Read the model definition and answer for the solid it produces. Units are mm, in the model's axes. A direction names the side the tool comes from. Give positions to 0.01 mm unless a question says otherwise; leave off trailing zeros. Order: outer loops, then holes, each group sorted by start corner. A loop starts at its lowest first (then second) coordinate and runs counter-clockwise, first axis right, second up. Notation, with made-up numbers: (-21.5, -18.75) - (-5.5, -18.75) arc R30 ccw to (-5.5, 12.25) - close; hole circle Ø5 at (84.5, 84.25). An arc over 180 degrees is marked (long way). Write each question's results on one line, items separated by ' | '. Start each with the question number.
Q1. A tool of negligible diameter and unlimited length cuts with its end or side. For faces 1 (the face through (-25, -3, 2)), 2 (the face through (37.5, 0, 31)), 3 (the face through (0, -22, 41)), from which of +Z, -Z, +X, -X, +Y, -Y can it reach the whole face along a straight path? Write none if from no direction.
Q2. Find section B-B on x = -7.5. Give the vertices of the cut face in (y, z).
Q3. For a pull along Y with two mould halves and no side action, classify faces 4 (the face through (25, -3, 2)), 5 (the face through (1, 25, 31)), 6 (the face through (-1, 17, 0)) as +Y half, -Y half, draft (parallel to the pull), parting line (faces both ways), or undercut.
Q4. Find section C-C on z = 60.5. Give the vertices of the cut face in (x, y), and give its area (3 significant figures).
Q5. Find section D-D on z = 70.5. Give the vertices of the cut face in (x, y), and give its area (4 significant figures).
Q6. Find the intervals of material crossed by line 1 along Y through (x, z) = (-14, 42); line 2 along X through (y, z) = (-12, 12); line 3 along Z through (x, y) = (-32.5, -18), in increasing order. Write a range as from..to.
Q7. Find section A-A on y = -4. Give the vertices of the cut face in (x, z), and give its area (3 significant figures).
Q8. A flat-ended cylindrical pin translates along its axis: P1, Ø1, axis at x = 16, y = 18, coming from the -Z side. Find the tip coordinate at first contact, or state that the pin passes through.
Solid Edge part; units mm, degrees
sketch "Sketch1" plane through (0, 0, 0) normal (0, 0, 1) x (1, 0, 0)
  line L0 (37.5, -25) -> (37.5, 25)
  line L1 (37.5, 25) -> (-37.5, 25)
  line L2 (-37.5, 25) -> (-37.5, -25)
  line L3 (-37.5, -25) -> (37.5, -25)
extrude "Protrusion1" add sketch "Sketch1" along normal blind 82
shell "Thinwall1" thickness 3 removed faces 1 at (-25.75, -16.1667, 82)
sketch "Sketch2" plane through (-37.5, 0, 30) normal (-1, 0, 0) x (0, -1, 0)
  line L0 (-25, 52) -> (-25, 32)
  line L1 (-25, 32) -> (25, 52)
  line L2 (25, 52) -> (-25, 52)
extrude "Cutout1" cut sketch "Sketch2" against normal blind 230
sketch "Sketch3" plane through (0, 0, 3) normal (0, 0, 1) x (1, 0, 0)
  line L0 (25, -15) -> (25, 15)
  line L1 (25, 15) -> (-25, 15)
  line L2 (-25, 15) -> (-25, -15)
  line L3 (-25, -15) -> (-25, -20.6045)
  line L4 (-25, -20.6045) -> (25, -20.6045)
  line L5 (25, -20.6045) -> (25, -15)
extrude "Cutout2" cut sketch "Sketch3" against normal blind 380
Working result:
1) face 1: +Z, -Z | face 2: +Z, -Z, +X, +Y, -Y | face 3: +Z
2) outline: (-25, 0) - (-20.6, 0) - (-20.6, 3) - (-22, 3) - (-22, 80.8) - (-25, 82) - close; (15, 0) - (25, 0) - (25, 62) - (22, 63.2) - (22, 3) - (15, 3) - close
3) face 4: undercut | face 5: +Y half | face 6: draft
4) outline: (-37.5, -25) - (37.5, -25) - (37.5, 25) - (-37.5, 25) - close; hole (-34.5, -22) - (34.5, -22) - (34.5, 22) - (-34.5, 22) - close | area: 714 mm²
5) outline: (-37.5, -25) - (37.5, -25) - (37.5, 3.75) - (34.5, 3.75) - (34.5, -22) - (-34.5, -22) - (-34.5, 3.75) - (-37.5, 3.75) - close | area: 379.5 mm²
6) line 1: -25..-22, 22..25 | line 2: -37.5..-34.5, 34.5..37.5 | line 3: 0..3
7) outline: (-37.5, 0) - (-25, 0) - (-25, 3) - (-34.5, 3) - (-34.5, 73.6) - (-37.5, 73.6) - close; (25, 0) - (37.5, 0) - (37.5, 73.6) - (34.5, 73.6) - (34.5, 3) - (25, 3) - close | area: 499 mm²
8) P1: z = 0
